Source: three-view drawing plus pictorial views. Frame: mm from the lowest corner of the part. A direction names the side the tool comes from. Give positions to 0.01 mm unless a question says otherwise; leave off trailing zeros. Write each loop counter-clockwise with the first axis right and the second up, starting at its lowest first coordinate (ties: lowest second). Pieces come first, ordered by that corner, then holes. Notation, with made-up numbers: M -33,15 L 23,15 A18 cw 23,40 Z; hole C 3.25,60.25 d1. An arc over 180 degrees is marked long. Return JSON: item names as keys, results as strings.
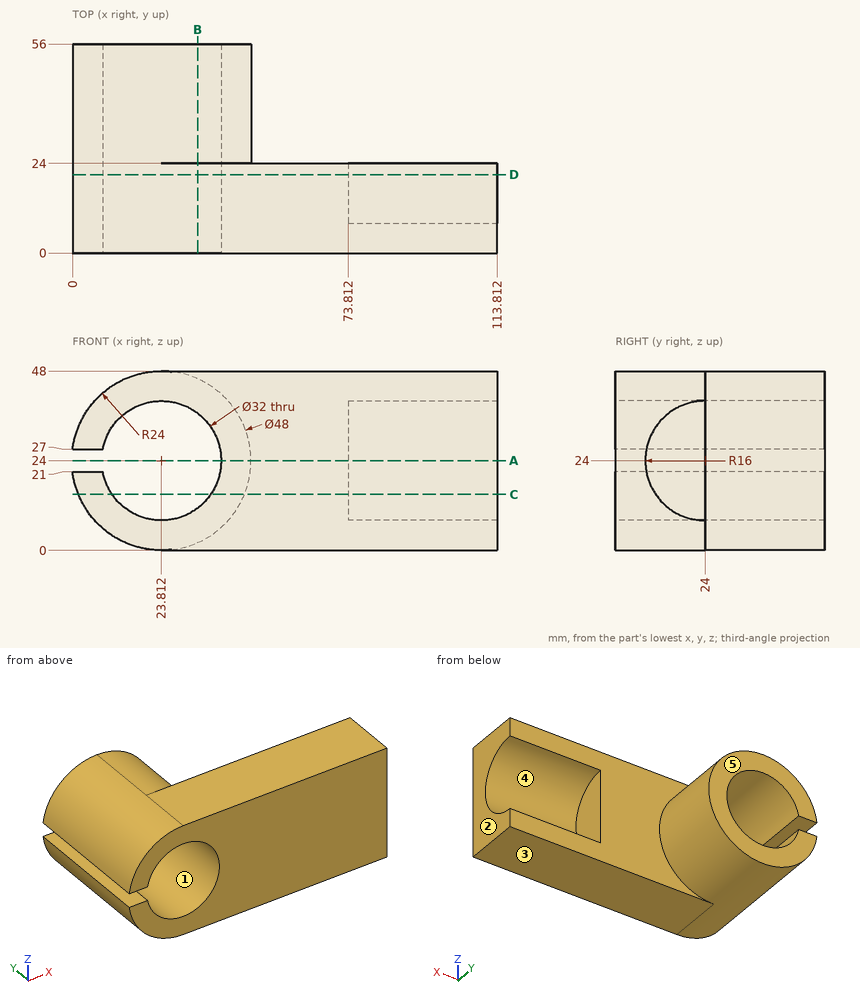
1) Cut plane C-C, the plane z = 15. Return the cut outline in (x, y), then the cut area to 3 significant figures.
Numbers:
{"outline": "M 1.56,0 L 10.58,0 L 10.58,56 L 1.56,56 Z; M 37.04,0 L 113.81,0 L 113.81,10.77 L 73.81,10.77 L 73.81,24 L 46.06,24 L 46.06,56 L 37.04,56 Z", "area": "2,110 mm²"}
2) Draft query along Z for the marked faces 1, 2 and 3. Return one class per face: released by +Z, released by -Z, zero draft, split by the parting line, or undercut.
Numbers:
{"face 1": "undercut", "face 2": "zero draft", "face 3": "released by -Z"}
3) Contact query for flat-ended pins moving along their axis: pin 1 Ø6.5 at (x, y) = (2, 24) entering from +Z; pin 2 Ø1.5 at (y, z) = (47.5, 41.5) entering from +X; pin 3 Ø1.5 at (y, z) = (32, 39) entering from +X. Output: stop coordinate, or through.
Numbers:
{"pin 1": "stops at z = 39.21", "pin 2": "stops at x = 41", "pin 3": "stops at x = 43.12"}
4) Set-up query: the marked faces 4 and 5. Return all of +Z, -Z, +X, -X, +Y, -Y with unobstructed straight access to the full face (end or side cutting, diameter ignored); none if empty.
Numbers:
{"face 4": "+X, +Y", "face 5": "+Z, -Z, +X, -X, +Y"}
5) Cut plane A-A, the plane z = 24. Return the cut outline in (x, y), then the cut area to 3 significant figures.
Numbers:
{"outline": "M 39.81,0 L 113.81,0 L 113.81,8 L 73.81,8 L 73.81,24 L 47.81,24 L 47.81,56 L 39.81,56 Z", "area": "1,390 mm²"}
6) Cut plane D-D, the plane y = 21. Return the cut outline in (x, z).
Numbers:
{"outline": "M 0,21 A24 ccw 23.81,0 L 113.81,0 L 113.81,8.28 L 73.81,8.28 L 73.81,39.72 L 113.81,39.72 L 113.81,48 L 23.81,48 A24 ccw 0,27 L 8.1,27 A16 cw long 8.1,21 Z"}
7) Cut plane B-B, the plane x = 33.5. Return the cut outline in (y, z).
Numbers:
{"outline": "M 0,0 L 24,0 L 24,2.04 L 56,2.04 L 56,11.27 L 0,11.27 Z; M 0,36.73 L 56,36.73 L 56,45.96 L 24,45.96 L 24,48 L 0,48 Z"}
8) Line query: line 1 (X direction, y = 26, z = 24); line 2 (X direction, y = 17.5, z = 37) (1 decimal); line 3 (Y direction, x = 108, z = 43). Output: solid intervals per line, ascending. Write a range as [from, to].
Numbers:
{"line 1": "x = [39.81, 47.81]", "line 2": "x = [3.6, 14.5], [33.1, 73.8]", "line 3": "y = [0, 24]"}
